from build123d import *

# Parameters (mm, degrees)
SKETCH2_R           = 2
BOSS_EXTRUDE1_DEPTH = 3
SKETCH5_R           = 2
CUT_EXTRUDE3_DEPTH  = 92
CUT_EXTRUDE5_DEPTH  = 10


with BuildPart() as part:
    # Sketch2 → Boss-Extrude1 (new body)
    with BuildSketch(Plane(origin=(0, 0, 0), x_dir=(1, 0, 0), z_dir=(0, 1, 0))):
        with BuildLine():
            Line((-242.852440467, 39.573874981), (-113.958962067, -159.70764714))
            ThreePointArc((-113.958962067, -159.70764714), (-103.371408315, -180.139975304), (-96.878813929, -202.217623429))
            ThreePointArc((-96.878813929, -202.217623429), (1.321917166, -283.333333333), (99.522648261, -202.217623429))
            ThreePointArc((99.522648261, -202.217623429), (106.015242647, -180.139975304), (116.6027964, -159.70764714))
            Line((116.6027964, -159.70764714), (244.060427664, 37.353919355))
            ThreePointArc((244.060427664, 37.353919355), (247.930993611, 139.46341826), (160.090354442, 191.668333333))
            Line((160.090354442, 191.668333333), (-160.090354442, 191.668333333))
            ThreePointArc((-160.090354442, 191.668333333), (-246.667324741, 140.214434267), (-242.852440467, 39.573874981))
        make_face()
        with Locations((-12.5, -192.545452)):
            Circle(SKETCH2_R, mode=Mode.SUBTRACT)
        with BuildLine():
            ThreePointArc((-55, -140), (-53.535533906, -136.464466094), (-50, -135))
            Line((-50, -135), (50, -135))
            ThreePointArc((50, -135), (53.535533906, -136.464466094), (55, -140))
            Line((55, -140), (55, -180))
            ThreePointArc((55, -180), (53.535533906, -183.535533906), (50, -185))
            Line((50, -185), (-50, -185))
            ThreePointArc((-50, -185), (-53.535533906, -183.535533906), (-55, -180))
            Line((-55, -180), (-55, -140))
        make_face(mode=Mode.SUBTRACT)
        with Locations((-12.5, -127)):
            Circle(SKETCH2_R, mode=Mode.SUBTRACT)
        with Locations((12.5, -192.545452)):
            Circle(SKETCH2_R, mode=Mode.SUBTRACT)
        with Locations((12.5, -127)):
            Circle(SKETCH2_R, mode=Mode.SUBTRACT)
        with Locations((-137.885861375, 65.174682453)):
            Circle(SKETCH2_R, mode=Mode.SUBTRACT)
        with Locations((-194.64988791, 97.947408453)):
            Circle(SKETCH2_R, mode=Mode.SUBTRACT)
        with BuildLine():
            Line((-113.564064606, 123.301270189), (-138.564064606, 80))
            Line((-138.564064606, 80), (-163.564064606, 36.698729811))
            ThreePointArc((-163.564064606, 36.698729811), (-166.600096399, 34.369100679), (-170.394191624, 34.868602792))
            Line((-170.394191624, 34.868602792), (-205.035207776, 54.868602792))
            ThreePointArc((-205.035207776, 54.868602792), (-207.364836907, 57.904634585), (-206.865334795, 61.698729811))
            Line((-206.865334795, 61.698729811), (-156.865334795, 148.301270189))
            ThreePointArc((-156.865334795, 148.301270189), (-153.829303001, 150.630899321), (-150.035207776, 150.131397208))
            Line((-150.035207776, 150.131397208), (-115.394191624, 130.131397208))
            ThreePointArc((-115.394191624, 130.131397208), (-113.064562493, 127.095365415), (-113.564064606, 123.301270189))
        make_face(mode=Mode.SUBTRACT)
        with Locations((-182.14988791, 119.598043547)):
            Circle(SKETCH2_R, mode=Mode.SUBTRACT)
        with Locations((-125.385861375, 86.825317547)):
            Circle(SKETCH2_R, mode=Mode.SUBTRACT)
        with Locations((137.885861375, 65.174682453)):
            Circle(SKETCH2_R, mode=Mode.SUBTRACT)
        with Locations((125.385861375, 86.825317547)):
            Circle(SKETCH2_R, mode=Mode.SUBTRACT)
        with BuildLine():
            Line((163.564064606, 36.698729811), (138.564064606, 80))
            Line((138.564064606, 80), (113.564064606, 123.301270189))
            ThreePointArc((113.564064606, 123.301270189), (113.064562493, 127.095365415), (115.394191624, 130.131397208))
            Line((115.394191624, 130.131397208), (150.035207776, 150.131397208))
            ThreePointArc((150.035207776, 150.131397208), (153.829303001, 150.630899321), (156.865334795, 148.301270189))
            Line((156.865334795, 148.301270189), (206.865334795, 61.698729811))
            ThreePointArc((206.865334795, 61.698729811), (207.364836907, 57.904634585), (205.035207776, 54.868602792))
            Line((205.035207776, 54.868602792), (187.7146997, 44.868602792))
            Line((187.7146997, 44.868602792), (170.394191624, 34.868602792))
            ThreePointArc((170.394191624, 34.868602792), (166.600096399, 34.369100679), (163.564064606, 36.698729811))
        make_face(mode=Mode.SUBTRACT)
        with Locations((194.64988791, 97.947408453)):
            Circle(SKETCH2_R, mode=Mode.SUBTRACT)
        with Locations((182.14988791, 119.598043547)):
            Circle(SKETCH2_R, mode=Mode.SUBTRACT)
    extrude(amount=BOSS_EXTRUDE1_DEPTH)

    # Sketch5 → Cut-Extrude3 (cut)
    with BuildSketch(Plane(origin=(0, 3, 0), x_dir=(1, 0, 0), z_dir=(0, 1, 0))):
        with Locations((0, 180.168332775)):
            Circle(SKETCH5_R)
        with Locations((236.5079546, 133.966482848)):
            Circle(SKETCH5_R)
        with Locations((-236.507954462, 133.966482869)):
            Circle(SKETCH5_R)
        with Locations((0, -271.833334923)):
            Circle(SKETCH5_R)
    extrude(amount=-CUT_EXTRUDE3_DEPTH, mode=Mode.SUBTRACT)

    # Sketch7 → Cut-Extrude5 (cut)
    with BuildSketch(Plane(origin=(0, 3, 0), x_dir=(1, 0, 0), z_dir=(0, 1, 0))):
        with BuildLine():
            Line((-1, 110.502325279), (-1, 105.502325279))
            ThreePointArc((-1, 105.502325279), (0, 104.502325279), (1, 105.502325279))
            Line((1, 105.502325279), (1, 110.502325279))
            ThreePointArc((1, 110.502325279), (0, 111.502325279), (-1, 110.502325279))
        make_face()
        with BuildLine():
            Line((-106.234238689, -40.545808051), (-103.734238689, -44.87593507))
            ThreePointArc((-103.734238689, -44.87593507), (-102.368213267, -45.241960479), (-102.002187858, -43.875935056))
            Line((-102.002187858, -43.875935056), (-104.502187858, -39.545808037))
            ThreePointArc((-104.502187858, -39.545808037), (-105.86821328, -39.179782628), (-106.234238689, -40.545808051))
        make_face()
        with BuildLine():
            Line((112.469526392, -63.7796108), (108.139399373, -61.2796108))
            ThreePointArc((108.139399373, -61.2796108), (106.773373969, -61.645636204), (107.139399373, -63.011661607))
            Line((107.139399373, -63.011661607), (111.469526392, -65.511661607))
            ThreePointArc((111.469526392, -65.511661607), (112.835551796, -65.145636204), (112.469526392, -63.7796108))
        make_face()
        with BuildLine():
            Line((85.622738875, -48.2796108), (81.292611856, -45.7796108))
            ThreePointArc((81.292611856, -45.7796108), (79.926586452, -46.145636204), (80.292611856, -47.511661607))
            Line((80.292611856, -47.511661607), (84.622738875, -50.011661607))
            ThreePointArc((84.622738875, -50.011661607), (85.988764279, -49.645636204), (85.622738875, -48.2796108))
        make_face()
        with BuildLine():
            Line((88.247094528, -71.734093472), (90.747094528, -67.403966453))
            ThreePointArc((90.747094528, -67.403966453), (90.381069124, -66.037941049), (89.01504372, -66.403966453))
            Line((89.01504372, -66.403966453), (86.51504372, -70.734093472))
            ThreePointArc((86.51504372, -70.734093472), (86.881069124, -72.100118875), (88.247094528, -71.734093472))
        make_face()
        with BuildLine():
            ThreePointArc((102.01504372, -43.887305954), (102.381069124, -45.253331358), (103.747094528, -44.887305954))
            Line((103.747094528, -44.887305954), (106.247094528, -40.557178935))
            ThreePointArc((106.247094528, -40.557178935), (105.881069124, -39.191153532), (104.51504372, -39.557178935))
            Line((104.51504372, -39.557178935), (102.01504372, -43.887305954))
        make_face()
        with BuildLine():
            ThreePointArc((-89.00218787, -66.392595562), (-90.368213274, -66.026570158), (-90.734238677, -67.392595562))
            Line((-90.734238677, -67.392595562), (-88.234238677, -71.72272258))
            ThreePointArc((-88.234238677, -71.72272258), (-86.868213274, -72.088747984), (-86.50218787, -70.72272258))
            Line((-86.50218787, -70.72272258), (-89.00218787, -66.392595562))
        make_face()
        with BuildLine():
            Line((-81.279756017, -45.768239915), (-85.609883036, -48.268239915))
            ThreePointArc((-85.609883036, -48.268239915), (-85.97590844, -49.634265319), (-84.609883036, -50.000290723))
            Line((-84.609883036, -50.000290723), (-80.279756017, -47.500290723))
            ThreePointArc((-80.279756017, -47.500290723), (-79.913730614, -46.134265319), (-81.279756017, -45.768239915))
        make_face()
        with BuildLine():
            ThreePointArc((-107.126543535, -63.000290723), (-106.760518131, -61.634265319), (-108.126543535, -61.268239915))
            Line((-108.126543535, -61.268239915), (-112.456670554, -63.768239915))
            ThreePointArc((-112.456670554, -63.768239915), (-112.822695957, -65.134265319), (-111.456670554, -65.500290723))
            Line((-111.456670554, -65.500290723), (-107.126543535, -63.000290723))
        make_face()
        with BuildLine():
            ThreePointArc((1, 79.502325279), (0, 80.502325279), (-1, 79.502325279))
            Line((-1, 79.502325279), (-1, 74.502325279))
            ThreePointArc((-1, 74.502325279), (0, 73.502325279), (1, 74.502325279))
            Line((1, 74.502325279), (1, 79.502325279))
        make_face()
        with BuildLine():
            Line((18, 93.502325279), (13, 93.502325279))
            ThreePointArc((13, 93.502325279), (12, 92.502325279), (13, 91.502325279))
            Line((13, 91.502325279), (18, 91.502325279))
            ThreePointArc((18, 91.502325279), (19, 92.502325279), (18, 93.502325279))
        make_face()
        with BuildLine():
            ThreePointArc((-13, 91.502325279), (-12, 92.502325279), (-13, 93.502325279))
            Line((-13, 93.502325279), (-18, 93.502325279))
            ThreePointArc((-18, 93.502325279), (-19, 92.502325279), (-18, 91.502325279))
            Line((-18, 91.502325279), (-13, 91.502325279))
        make_face()
    extrude(amount=-CUT_EXTRUDE5_DEPTH, mode=Mode.SUBTRACT)


solid = part.part
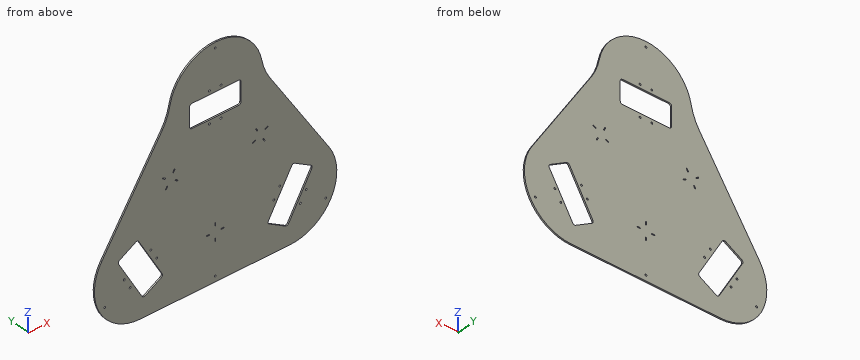
Work out the finished part from the listing and answer in its coordinate system (mm). Give positions to 0.01 mm unless a question says otherwise; leave off trailing zeros. Order: outer loops, then holes, each group sorted by start corner. A loop starts at its lowest first (then second) coordinate and runs counter-clockwise, first axis right, second up. Notation, with made-up numbers: (9, -12.75) - (54, -12.75) arc R20 cw to (54, 20.25) - close; hole circle Ø11 at (76, 77). An arc over 180 degrees is marked (long way). Answer as CSV lines item,"result". Start each with the question number.
Q1. Find the intervals of material crossed by L1, parallel to Z at x = 0, y = 0.85; L2, parallel to Z at x = -12.5, y = 1.45; L3, parallel to X at y = 0.5, z = 40, in increasing order. Write a range as [from, to].
Q2. The part is cut by section B-B (y = 2.25). Give the number of separate pieces and of enclosed holes in the cut face, then the cut area to 3 significant figures.
Q3. Given pin 1 Ø1.5 at (y, z) = (2, -78) entering from -X; pin 2 Ø2.5 at (x, z) = (-236.51, -133.97) entering from +Y; pin 3 Ø1.5 at (y, z) = (1.5, -108.5) entering from +X; pin 4 Ø0.9 at (y, z) = (1.5, 159) entering from +X, each flat-ended and moving along its own axis, determine where each tip first touches the part or whether it passes through.
Q4. The part is cut by section A-A (x = -29.5). Write down the section's boundary in (y, z), then the cut area to 3 significant figures.
Q5. The part is cut by section C-C (z = 1.5). Write down the section's boundary in (x, y).
Check result:
1,L1,"z = [-191.67, -182.17], [-178.17, -111.5], [-104.5, -80.5], [-73.5, 135], [185, 269.83], [273.83, 283.32]"
1,L2,"z = [-191.67, -93.37], [-91.64, 125], [129, 135], [185, 190.55], [194.55, 282.37]"
1,L3,"x = [-191.38, -106.37], [-104.24, 104.26], [106.38, 194.03]"
2,separate pieces,"1"
2,enclosed holes,"31"
2,area,"150,000 mm²"
3,pin 1,"stops at x = -257.6"
3,pin 2,"passes through"
3,pin 3,"stops at x = 258.79"
3,pin 4,"stops at x = 117.35"
4,outline,"(0, -191.67) - (3, -191.67) - (3, 135) - (0, 135) - close; (0, 185) - (3, 185) - (3, 278.46) - (0, 278.46) - close"
4,area,"1,260 mm²"
5,outline,"(-216.29, 0) - (218.93, 0) - (218.93, 3) - (-216.29, 3) - close"
